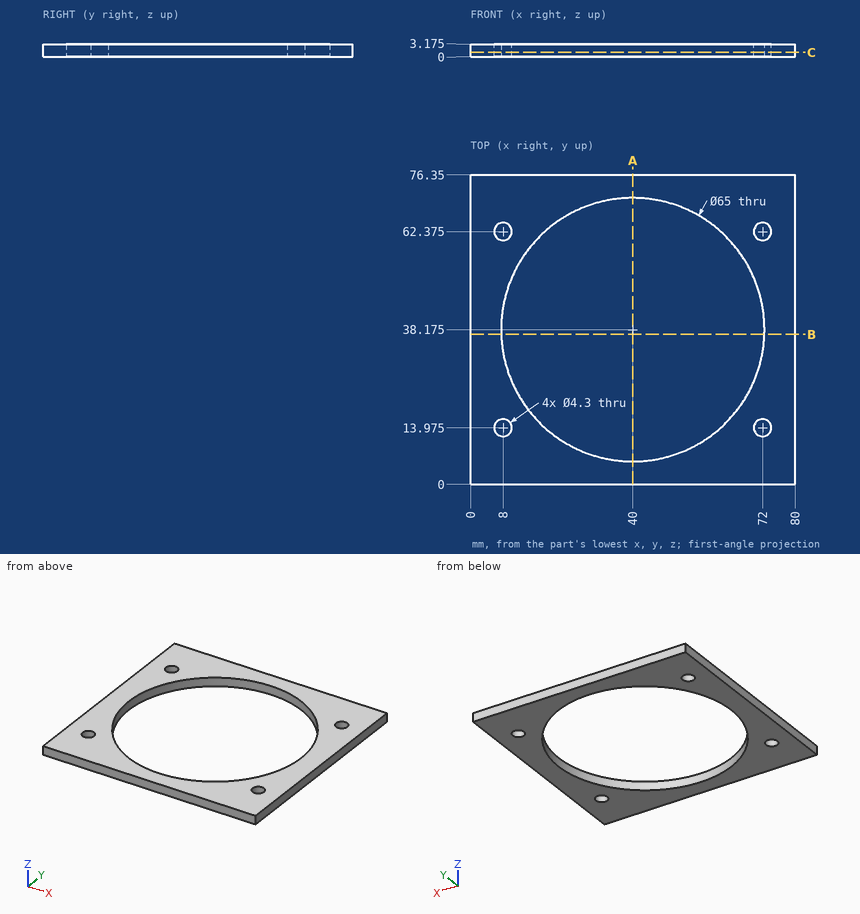
Input: dimensioned drawing with shaded views. Units: mm. Origin: part minimum x, y, z. Give positions to 0.01 mm unless a question says otherwise; leave off trailing zeros. Write each loop counter-clockwise with the first axis right and the second up, starting at its lowest first coordinate (ties: lowest second). Pieces come first, ordered by that corner, then holes. Notation, with made-up numbers: M 45.5,36 L 87.5,36 A21 cw 87.5,72 Z; hole C 24.5,-24 d6. An arc over 180 degrees is marked long. Write item = value, one per line. Start each with the question number.
1) Cut plane B-B on y = 37. Return the cut outline in (x, z) (3 decimals), then the cut area to 3 significant figures.
2) Cut plane A-A on x = 40. Return the cut outline in (y, z) (3 decimals).
3) Cut plane C-C on z = 1.1. Return the cut outline in (x, y) (3 decimals), then the cut area to 3 significant figures.
4) Material intervals for line 1 along X through (y, z) = (39, 0.85); line 2 along X through (y, z) = (63, 0.45); line 3 along X through (y, z) = (41, 0.5), sorted ascending. Write a range as [from, to].
Solved:
q1.outline = M 0,0 L 7.521,0 L 7.521,3.175 L 0,3.175 Z; M 72.479,0 L 80,0 L 80,3.175 L 72.479,3.175 Z
q1.area = 47.8 mm2
q2.outline = M 0,0 L 5.675,0 L 5.675,3.175 L 0,3.175 Z; M 70.675,0 L 76.35,0 L 76.35,3.175 L 70.675,3.175 Z
q3.outline = M 0,0 L 80,0 L 80,76.35 L 0,76.35 Z; hole C 8,13.975 d4.3; hole C 8,62.375 d4.3; hole C 40,38.175 d65; hole C 72,13.975 d4.3; hole C 72,62.375 d4.3
q3.area = 2,730 mm2
q4.line_1 = [0, 7.51], [72.49, 80]
q4.line_2 = [0, 5.94], [10.06, 19.02], [60.98, 69.94], [74.06, 80]
q4.line_3 = [0, 7.62], [72.38, 80]
